The drawing under review shows one solid part. Ordinate dimensions are in mm from its lowest x, y, z. Coordinates: 2 decimals unless noted, no trailing zeros. Order: outer loops, then holes, each group sorted by start corner. A loop starts at its lowest first (then second) coordinate and runs counter-clockwise, first axis right, second up. Notation, with made-up numbers: (39, -14) -> (48, -14) arc R25 cw to (48, 21) -> close; hole circle Ø4 at (82, 10.5). An arc over 180 degrees is marked (long way). Use one line per item in the form item = value.
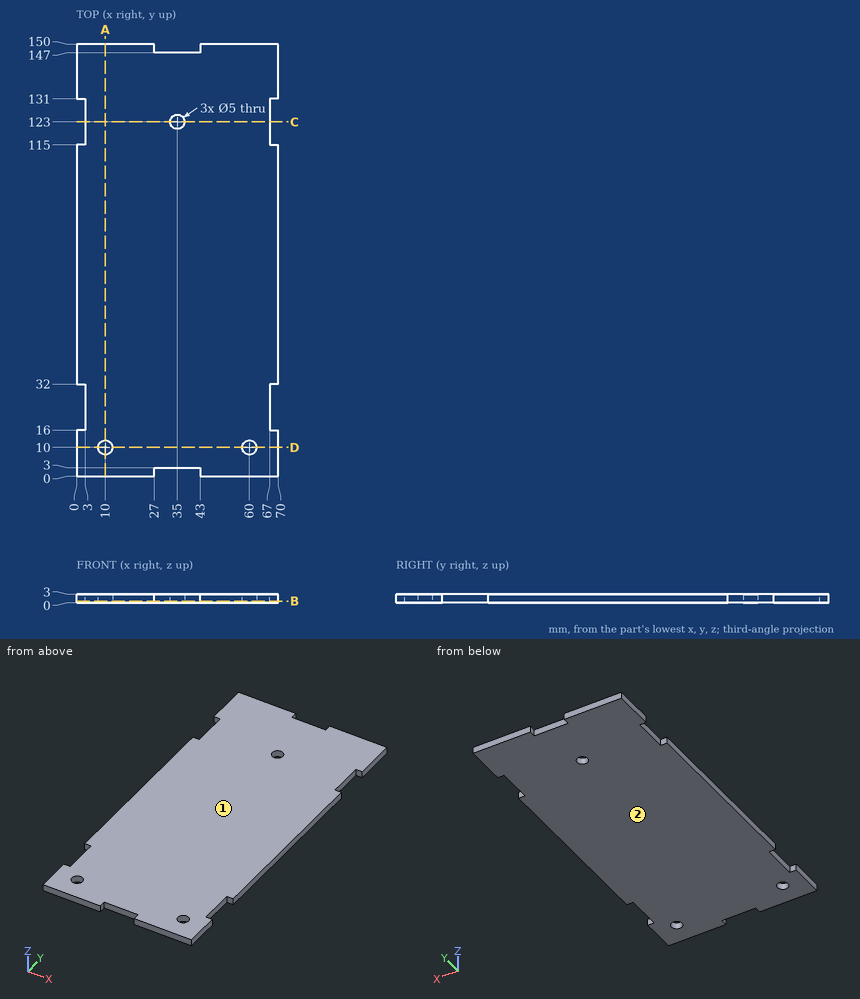
Item 1: We need section D-D (y = 10). Write out the cut boundary in (x, z).
Results found:
outline = (0, 0) -> (7.5, 0) -> (7.5, 3) -> (0, 3) -> close; (12.5, 0) -> (57.5, 0) -> (57.5, 3) -> (12.5, 3) -> close; (62.5, 0) -> (70, 0) -> (70, 3) -> (62.5, 3) -> close
Item 2: We need section A-A (x = 10). Write out the cut boundary in (y, z).
Results found:
outline = (0, 0) -> (7.5, 0) -> (7.5, 3) -> (0, 3) -> close; (12.5, 0) -> (150, 0) -> (150, 3) -> (12.5, 3) -> close
Item 3: Draft analysis for pull direction Z (two halves, no side actions). For the marked faces 1 and 2, state which applies: released by +Z, released by -Z, zero draft, split by the parting line, or undercut.
Results found:
face_1 = released by +Z
face_2 = released by -Z
Item 4: To check wall thickness, follow L1, parallel to Y at x = 60, z = 1.65; L2, parallel to Y at x = 35, z = 1.35; L3, parallel to Y at x = 28, z = 0.3. State the ranges of each line that lie inside material, in increasing order. Write a range as from..to.
Results found:
L1 = 0..7.5, 12.5..150
L2 = 3..120.5, 125.5..147
L3 = 3..147
Item 5: Clearance check with flat-ended pins moving along their axes: pin 1 (0.9 mm diameter, centred on y = 23, z = 1, fed in from -X); pin 2 (0.9 mm diameter, centred on y = 121, z = 1.5, fed in from +X); pin 3 (4.5 mm diameter, centred on x = 10, y = 10, fed in from -Z). State where each tip first meets the part, or that it passes through.
Results found:
pin_1 = 3
pin_2 = 67
pin_3 = through
Item 6: We need section C-C (y = 123). Write out the cut boundary in (x, z), plus the area to 3 significant figures.
Results found:
outline = (3, 0) -> (32.5, 0) -> (32.5, 3) -> (3, 3) -> close; (37.5, 0) -> (67, 0) -> (67, 3) -> (37.5, 3) -> close
area = 177 mm²
Item 7: We need section B-B (z = 0.65). State how many separate pieces and enclosed holes the cut face has, plus the area to 3 significant figures.
Results found:
separate_pieces = 1
enclosed_holes = 3
area = 10,200 mm²
